For this review, take the finished solid that the model builds, in its own axes (mm). Face numbers are marked on the shaded views. Round coordinates to 2 decimals unless told otherwise and drop trailing zeros. Write each loop counter-clockwise with the first axis right and the second up, starting at its lowest first coordinate (ties: lowest second). Pieces come first, ordered by that corner, then holes. Notation, with made-up numbers: M 69,75.25 L 79,75.25 A18 cw 79,95.25 Z; hole C 66,17 d10. An arc over 180 degrees is marked long. Answer in a Markdown table with one row per item.
```python
from build123d import *

# Parameters (mm, degrees)
SKETCH1_W           = 66.4
SKETCH1_H           = 5.8
BOSS_EXTRUDE1_DEPTH = 25
SKETCH2_R           = 8.875
CUT_EXTRUDE1_DEPTH  = 6.8
CUT_EXTRUDE2_DEPTH  = 6.8


with BuildPart() as part:
    # Sketch1 → Boss-Extrude1 (new body)
    with BuildSketch(Plane.XY):
        with Locations((0, 59.6)):
            Rectangle(SKETCH1_W, SKETCH1_H)
    extrude(amount=BOSS_EXTRUDE1_DEPTH)

    # Sketch2 → Cut-Extrude1 (cut, through all)
    with BuildSketch(Plane(origin=(0, 62.5, 0), x_dir=(1, 0, 0), z_dir=(0, 1, 0))):
        with Locations((0, -12.500000019)):
            Circle(SKETCH2_R)
    extrude(amount=-CUT_EXTRUDE1_DEPTH, mode=Mode.SUBTRACT)

    # Sketch3 → Cut-Extrude2 (cut, through all)
    with BuildSketch(Plane.XZ.offset(-56.7)):
        with BuildLine():
            Line((-1.2, 3.706501), (1.2, 3.706501))
            Line((1.2, 3.706501), (1.2, 2.657885155))
            ThreePointArc((1.2, 2.657885155), (0, 2.585000019), (-1.2, 2.657885155))
            Line((-1.2, 2.657885155), (-1.2, 3.706501))
        make_face()
    extrude(amount=-CUT_EXTRUDE2_DEPTH, mode=Mode.SUBTRACT)


solid = part.part
```
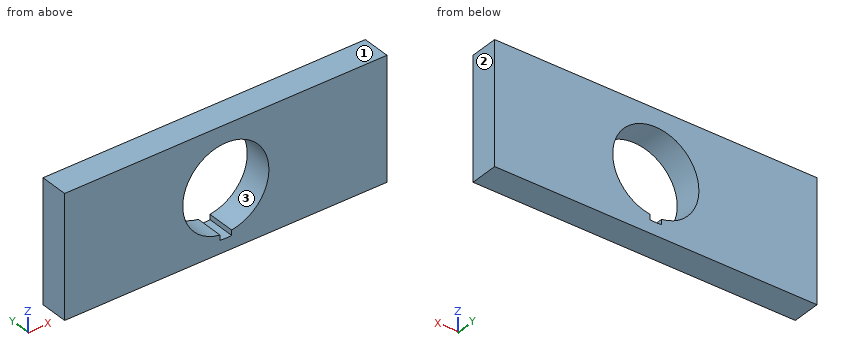
Q1. Take a section at A-A (x = 0). State the section outline as (y, z) points (3 decimals).
Found:
| item | result |
|---|---|
| outline | M 56.7,0 L 62.5,0 L 62.5,2.585 L 56.7,2.585 Z; M 56.7,21.375 L 62.5,21.375 L 62.5,25 L 56.7,25 Z |
Q2. Mouldability with a two-part tool opening along X and no side actions: class the marked faces 1, 2 and 3 as +X half, -X half, draft (parallel to the pull), parting line (faces both ways), or undercut.
Found:
| item | result |
|---|---|
| face 1 | draft |
| face 2 | +X half |
| face 3 | undercut |
Q3. For probe 1 along X at (y, z) = (62.05, 12); probe 2 along Z at (x, y) = (0, 58.5) (3 decimals); probe 3 along X at (y, z) = (57.2, 3.25), list the stretches that pass through material, from the lowest coordinate up.
Found:
| item | result |
|---|---|
| probe 1 | -33.2 to -8.86, 8.86 to 33.2 |
| probe 2 | 0 to 2.585, 21.375 to 25 |
| probe 3 | -33.2 to -1.2, 1.2 to 33.2 |
Q4. Insertion check: P1, Ø8, axis at x = -3.5, z = 9.5, coming from the +Y side; P2, Ø1, axis at x = -9, y = 57.5, coming from the -Z side. Each pin has a flat end and moves straight along its axis. Give the tip position at first contact, or say it passes through.
Found:
| item | result |
|---|---|
| P1 | through |
| P2 | z = 0 |
Q5. Take a section at B-B (z = 12.5). State the section outline as (x, y) points (3 decimals), then the cut area to 3 significant figures.
Found:
| item | result |
|---|---|
| outline | M -33.2,56.7 L -8.875,56.7 L -8.875,62.5 L -33.2,62.5 Z; M 8.875,56.7 L 33.2,56.7 L 33.2,62.5 L 8.875,62.5 Z |
| area | 282 mm² |
